from build123d import *

# Parameters (mm, degrees)
SKETCH_1_R          = 1.6
EXTRUDE_1_DEPTH     = 4
SKETCH_2_R          = 1.6
CUT_EXTRUDE_1_DEPTH = 10
FILLET_1_R          = 3


with BuildPart() as part:
    # 草图1 → 凸台-拉伸1 (new body)
    with BuildSketch(Plane(origin=(0, 0, 0), x_dir=(1, 0, 0), z_dir=(0, 1, 0))):
        with BuildLine():
            Line((-26.580295873, 0), (-26.580295873, -68.504426064))
            Line((-26.580295873, -68.504426064), (26.580295873, -68.504426064))
            Line((26.580295873, -68.504426064), (26.580295873, 0))
            ThreePointArc((26.580295873, 0), (0, 26.580295873), (-26.580295873, 0))
        make_face()
        with Locations(Location((17, 0, 0), (0, 0, 270))):
            Circle(SKETCH_1_R, mode=Mode.SUBTRACT)
        with Locations(Location((-17, 0, 0), (0, 0, 90))):
            Circle(SKETCH_1_R, mode=Mode.SUBTRACT)
        with Locations(Location((0, 17, 0), (0, 0, 270))):
            Circle(SKETCH_1_R, mode=Mode.SUBTRACT)
        with Locations(Location((0, -17, 0), (0, 0, 270))):
            Circle(SKETCH_1_R, mode=Mode.SUBTRACT)
        with BuildLine():
            Line((-14.695026261, 13.713220631), (-6.515150502, 19.014728906))
            ThreePointArc((-6.515150502, 19.014728906), (-2.694610628, 17.158059668), (-4.560612538, 13.342069303))
            ThreePointArc((-4.560612538, 13.342069303), (0, 14.1), (4.560612538, 13.342069303))
            ThreePointArc((4.560612538, 13.342069303), (2.694610628, 17.158059668), (6.515150502, 19.014728906))
            Line((6.515150502, 19.014728906), (13.857784146, 14.558867106))
            ThreePointArc((13.857784146, 14.558867106), (13.927445578, 10.331314347), (9.700465883, 10.232837419))
            ThreePointArc((9.700465883, 10.232837419), (0.41557213, -14.093874549), (-10.286539783, 9.643500365))
            ThreePointArc((-10.286539783, 9.643500365), (-14.510070274, 9.490986437), (-14.695026261, 13.713220631))
        make_face(mode=Mode.SUBTRACT)
    extrude(amount=EXTRUDE_1_DEPTH)

    # 草图2 → 切除-拉伸1 (cut)
    with BuildSketch(Plane.XZ):
        with Locations(Location((21.580295873, 63.504426064, 0), (0, 0, 270))):
            Circle(SKETCH_2_R)
        with Locations(Location((13.580295873, 63.504426064, 0), (0, 0, 270))):
            Circle(SKETCH_2_R)
        with Locations(Location((-13.580295873, 63.504426064, 0), (0, 0, 270))):
            Circle(SKETCH_2_R)
        with Locations(Location((-21.580295873, 63.504426064, 0), (0, 0, 270))):
            Circle(SKETCH_2_R)
    extrude(amount=-CUT_EXTRUDE_1_DEPTH, mode=Mode.SUBTRACT)

    # 圆角1
    fillet_1_edges = [part.edges().sort_by_distance(p)[0] for p in [
        (-26.580295873, 2, 68.504426064),
        (26.580295873, 2, 68.504426064),
    ]]
    fillet(fillet_1_edges, radius=FILLET_1_R)


solid = part.part
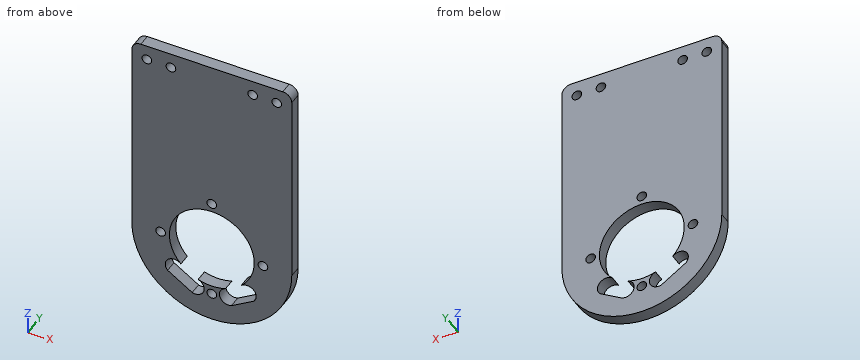
Model file for the job. Use its own axes, mm. Give positions to 0.01 mm unless a question says otherwise; leave off trailing zeros. Loops run counter-clockwise (first coordinate to the right, second up) from the corner with the lowest first, then second, coordinate; pieces in that order, holes last. Notation, with made-up numbers: (3, -12) -> (62, -12) arc R28 cw to (62, 25) -> close; hole circle Ø9 at (-3, 22.5). An arc over 180 degrees is marked (long way). Use a Markdown table: item, result. Add a question column.
(1) Drop a flat-ended pin along its axis: pin 1 Ø1 at (x, y) = (-18, 0.5) entering from -Z. Give the stop position or say it passes through.
(2) Slice it at D-D on z = -17. List the corners of the cut face in (x, y).
(3) Wall check: line 1 along Z through (x, y) = (-11, 0.4); line 2 along X through (y, z) = (2.9, -17); line 3 along Z through (x, y) = (-17, 1.9). Give the ranges that are in metal, low to high.
(4) Slice it at B-B on x = 0. List the corners of the cut face in (y, z).
(5) Slice it at A-A on z = 17. List the corners of the cut face in (x, y), and give its area (3 significant figures).
(6) Slice it at C-C on y = 3.1. Give the number of separate pieces and of enclosed holes in the cut face, and give its area (3 significant figures).
Filled sheet:
| question | item | result |
|---|---|---|
| 1 | pin 1 | z = -20.01 |
| 2 | outline | (-20.43, 0) -> (-9.62, 0) -> (-9.62, 4) -> (-20.43, 4) -> close; (-2.64, 0) -> (-1.6, 0) -> (-1.6, 4) -> (-2.64, 4) -> close; (1.6, 0) -> (2.64, 0) -> (2.64, 4) -> (1.6, 4) -> close; (9.84, 0) -> (20.43, 0) -> (20.43, 4) -> (9.84, 4) -> close |
| 3 | line 1 | -24.2 to -16.11, -9.08 to -8.82, 8.82 to 68.5 |
| 3 | line 2 | -20.43 to -9.62, -2.64 to -1.6, 1.6 to 2.64, 9.84 to 20.43 |
| 3 | line 3 | -20.43 to -1.6, 1.6 to 68.5 |
| 4 | outline | (0, -26.58) -> (4, -26.58) -> (4, -18.6) -> (0, -18.6) -> close; (0, -15.4) -> (4, -15.4) -> (4, -14.1) -> (0, -14.1) -> close; (0, 14.1) -> (4, 14.1) -> (4, 15.4) -> (0, 15.4) -> close; (0, 18.6) -> (4, 18.6) -> (4, 68.5) -> (0, 68.5) -> close |
| 5 | outline | (-26.58, 0) -> (-1.6, 0) -> (-1.6, 4) -> (-26.58, 4) -> close; (1.6, 0) -> (26.58, 0) -> (26.58, 4) -> (1.6, 4) -> close |
| 5 | area | 200 mm2 |
| 6 | separate pieces | 1 |
| 6 | enclosed holes | 9 |
| 6 | area | 3,910 mm2 |
